```python
from build123d import *

# Parameters (mm, degrees)
SKETCH1_R           = 1.6
BOSS_EXTRUDE1_DEPTH = 4
FILLET1_R           = 5


with BuildPart() as part:
    # Sketch1 → Boss-Extrude1 (new body)
    with BuildSketch(Plane(origin=(0, 0, 0), x_dir=(1, 0, 0), z_dir=(0, 1, 0))):
        Polygon((-50, -50), (50, -50), (50, 50), (12.5, 50), (12.5, 40), (-12.5, 40), (-12.5, 50), (-50, 50), align=None)
        with Locations((-45, -45)):
            Circle(SKETCH1_R, mode=Mode.SUBTRACT)
        with Locations((-25, -25.66)):
            Circle(SKETCH1_R, mode=Mode.SUBTRACT)
        with Locations((-12.5, -16)):
            Circle(SKETCH1_R, mode=Mode.SUBTRACT)
        with Locations((0, -25.66)):
            Circle(SKETCH1_R, mode=Mode.SUBTRACT)
        with Locations((45, -45)):
            Circle(SKETCH1_R, mode=Mode.SUBTRACT)
        with Locations((25, -25.66)):
            Circle(SKETCH1_R, mode=Mode.SUBTRACT)
        with Locations((12.5, -16)):
            Circle(SKETCH1_R, mode=Mode.SUBTRACT)
        with Locations((-25, 17.66)):
            Circle(SKETCH1_R, mode=Mode.SUBTRACT)
        with Locations((-45, 45)):
            Circle(SKETCH1_R, mode=Mode.SUBTRACT)
        with Locations((0, 17.66)):
            Circle(SKETCH1_R, mode=Mode.SUBTRACT)
        with Locations((25, 17.66)):
            Circle(SKETCH1_R, mode=Mode.SUBTRACT)
        with Locations((45, 45)):
            Circle(SKETCH1_R, mode=Mode.SUBTRACT)
    extrude(amount=BOSS_EXTRUDE1_DEPTH)

    # Fillet1
    fillet1_edges = [part.edges().sort_by_distance(p)[0] for p in [
        (50, 2, -50),
        (50, 2, 50),
        (-50, 2, 50),
        (-50, 2, -50),
    ]]
    fillet(fillet1_edges, radius=FILLET1_R)


solid = part.part
```
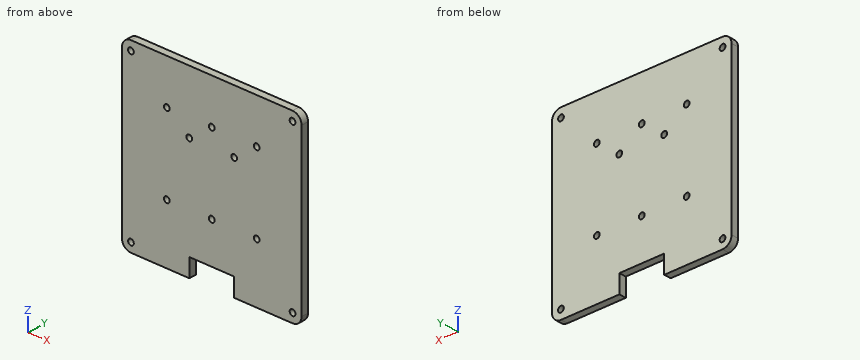
Verification items for the finished model (mm, model axes). Give positions to 0.01 mm unless a question says otherwise; leave off trailing zeros. Order: outer loops, then holes, each group sorted by start corner. A loop starts at its lowest first (then second) coordinate and runs counter-clockwise, first axis right, second up. Notation, with made-up numbers: (71.5, 18) -> (84.5, 18) arc R26 ccw to (84.5, 33) -> close; hole circle Ø10 at (78.5, 53.25). An arc over 180 degrees is marked (long way). One line per item, written item: value.
(1) Sectioned sample at D-D on z = -41.5. Record the cut outline in (x, y), then the cut area to 3 significant figures.
Final values:
outline: (-50, 0) -> (-12.5, 0) -> (-12.5, 4) -> (-50, 4) -> close; (12.5, 0) -> (50, 0) -> (50, 4) -> (12.5, 4) -> close
area: 300 mm^2
(2) Scan lines: line 1 along X through (y, z) = (2.2, 25.66); line 2 along Z through (x, y) = (45, 1.8). Record each from-to range of solid material in increasing order. Write a range as [from, to].
Final values:
line 1: [-50, -26.6], [-23.4, -1.6], [1.6, 23.4], [26.6, 50]
line 2: [-50, -46.6], [-43.4, 43.4], [46.6, 50]
(3) Sectioned sample at C-C on z = -17.66. Record the cut outline in (x, y).
Final values:
outline: (-50, 0) -> (-26.6, 0) -> (-26.6, 4) -> (-50, 4) -> close; (-23.4, 0) -> (-1.6, 0) -> (-1.6, 4) -> (-23.4, 4) -> close; (1.6, 0) -> (23.4, 0) -> (23.4, 4) -> (1.6, 4) -> close; (26.6, 0) -> (50, 0) -> (50, 4) -> (26.6, 4) -> close
(4) Sectioned sample at B-B on y = 0.95. Count the separate pieces of the cut face and the enclosed holes in it, then the cut area to 3 significant figures.
Final values:
separate pieces: 1
enclosed holes: 12
area: 9,630 mm^2
(5) Sectioned sample at A-A on x = 25. Record the cut outline in (y, z).
Final values:
outline: (0, -50) -> (4, -50) -> (4, -19.26) -> (0, -19.26) -> close; (0, -16.06) -> (4, -16.06) -> (4, 24.06) -> (0, 24.06) -> close; (0, 27.26) -> (4, 27.26) -> (4, 50) -> (0, 50) -> close
